Model file for the job. Use its own axes, mm. A direction names the side the tool comes from. Give positions to 0.01 mm unless a question says otherwise; leave off trailing zeros. Loops run counter-clockwise (first coordinate to the right, second up) from the corner with the lowest first, then second, coordinate; pieces in that order, holes last. Notation, with made-up numbers: M 47.25,12 L 52.25,12 A36 ccw 52.25,51 Z; hole C 55.25,84 d9. An arc over 180 degrees is marked long. Answer in a Markdown table with one row per item.
```python
from build123d import *

# Parameters (mm, degrees)
SKETCH1_R           = 173.85
SKETCH1_R_2         = 126.85
SKETCH1_R_3         = 4.1
BOSS_EXTRUDE1_DEPTH = 5
SKETCH1_3_R         = 146.85
SKETCH1_3_R_2       = 144.85
SKETCH1_3_R_3       = 126.85
BOSS_EXTRUDE2_DEPTH = 30
CUT_EXTRUDE1_START  = 9.5
SKETCH1_4_R         = 146.85
SKETCH1_4_R_2       = 144.85
CUT_EXTRUDE1_DEPTH  = 2.5
CUT_EXTRUDE2_START  = 21.5
SKETCH1_5_R         = 146.85
SKETCH1_5_R_2       = 144.85
CUT_EXTRUDE2_DEPTH  = 2.5


with BuildPart() as part:
    # Sketch1 → Boss-Extrude1 (new body)
    with BuildSketch(Plane(origin=(0, 0, 0), x_dir=(1, 0, 0), z_dir=(0, 1, 0))):
        with Locations(Location((0, 0, 0), (0, 0, 270))):
            Circle(SKETCH1_R)
        with Locations(Location((0, 0, 0), (0, 0, 270))):
            Circle(SKETCH1_R_2, mode=Mode.SUBTRACT)
        with Locations(Location((0, 161.925, 0), (0, 0, 270))):
            Circle(SKETCH1_R_3, mode=Mode.SUBTRACT)
        with Locations(Location((140.231163508, 80.9625, 0), (0, 0, 270))):
            Circle(SKETCH1_R_3, mode=Mode.SUBTRACT)
        with Locations(Location((140.231163508, -80.9625, 0), (0, 0, 270))):
            Circle(SKETCH1_R_3, mode=Mode.SUBTRACT)
        with Locations(Location((0, -161.925, 0), (0, 0, 270))):
            Circle(SKETCH1_R_3, mode=Mode.SUBTRACT)
        with Locations(Location((-140.231163508, -80.9625, 0), (0, 0, 270))):
            Circle(SKETCH1_R_3, mode=Mode.SUBTRACT)
        with Locations(Location((-140.231163508, 80.9625, 0), (0, 0, 270))):
            Circle(SKETCH1_R_3, mode=Mode.SUBTRACT)
    extrude(amount=BOSS_EXTRUDE1_DEPTH)

    # Sketch1_3 → Boss-Extrude2 (add)
    # profile 1 of 2: a face of its own
    with BuildSketch(Plane(origin=(0, 0, 0), x_dir=(1, 0, 0), z_dir=(0, 1, 0))):
        with Locations(Location((0, 0, 0), (0, 0, 270))):
            Circle(SKETCH1_3_R)
        Circle(SKETCH1_3_R_2, mode=Mode.SUBTRACT)
    # profile 2 of 2: a face of its own
    with BuildSketch(Plane(origin=(0, 0, 0), x_dir=(1, 0, 0), z_dir=(0, 1, 0))):
        Circle(SKETCH1_3_R_2)
        with Locations(Location((0, 0, 0), (0, 0, 270))):
            Circle(SKETCH1_3_R_3, mode=Mode.SUBTRACT)
    extrude(amount=BOSS_EXTRUDE2_DEPTH)

    # Sketch1_4 → Cut-Extrude1 (cut)
    with BuildSketch(Plane(origin=(0, 0, 0), x_dir=(1, 0, 0), z_dir=(0, 1, 0)).offset(CUT_EXTRUDE1_START)):
        with Locations(Location((0, 0, 0), (0, 0, 270))):
            Circle(SKETCH1_4_R)
        with Locations(Location((0, 0, 0), (0, 0, 270))):
            Circle(SKETCH1_4_R_2, mode=Mode.SUBTRACT)
    extrude(amount=CUT_EXTRUDE1_DEPTH, mode=Mode.SUBTRACT)

    # Sketch1_5 → Cut-Extrude2 (cut)
    with BuildSketch(Plane(origin=(0, 0, 0), x_dir=(1, 0, 0), z_dir=(0, 1, 0)).offset(CUT_EXTRUDE2_START)):
        with Locations(Location((0, 0, 0), (0, 0, 270))):
            Circle(SKETCH1_5_R)
        with Locations(Location((0, 0, 0), (0, 0, 270))):
            Circle(SKETCH1_5_R_2, mode=Mode.SUBTRACT)
    extrude(amount=CUT_EXTRUDE2_DEPTH, mode=Mode.SUBTRACT)


solid = part.part
```
(1) Saw through at B-B, the plane x = -43.5. Give the cut face in (y, z), and give its area (3 significant figures).
Established:
| item | result |
|---|---|
| outline | M 0,-168.32 L 5,-168.32 L 5,-140.26 L 9.5,-140.26 L 9.5,-138.16 L 12,-138.16 L 12,-140.26 L 21.5,-140.26 L 21.5,-138.16 L 24,-138.16 L 24,-140.26 L 30,-140.26 L 30,-119.16 L 0,-119.16 Z; M 0,119.16 L 30,119.16 L 30,140.26 L 24,140.26 L 24,138.16 L 21.5,138.16 L 21.5,140.26 L 12,140.26 L 12,138.16 L 9.5,138.16 L 9.5,140.26 L 5,140.26 L 5,168.32 L 0,168.32 Z |
| area | 1,530 mm2 |
(2) Saw through at A-A, the plane z = 0. Give the cut face in (x, y).
Established:
| item | result |
|---|---|
| outline | M -173.85,0 L -126.85,0 L -126.85,30 L -146.85,30 L -146.85,24 L -144.85,24 L -144.85,21.5 L -146.85,21.5 L -146.85,12 L -144.85,12 L -144.85,9.5 L -146.85,9.5 L -146.85,5 L -173.85,5 Z; M 126.85,0 L 173.85,0 L 173.85,5 L 146.85,5 L 146.85,9.5 L 144.85,9.5 L 144.85,12 L 146.85,12 L 146.85,21.5 L 144.85,21.5 L 144.85,24 L 146.85,24 L 146.85,30 L 126.85,30 Z |
(3) Mould opens along X. For faces 1 (the cylindrical face through (44.11, 7.22, 140.07)), 2 (the flat face through (-109.5, 30, 64.6)), 3 (the cylindrical face through (141.46, 2.46, -77.05)) say: pulls with the +X half, pulls with the -X half, needs draft (parallel to the pull), parting line crosses it, or undercut.
Established:
| item | result |
|---|---|
| face 1 | parting line crosses it |
| face 2 | needs draft |
| face 3 | undercut |
(4) Flat gauge pins, fed straight in: P1, Ø2, axis at y = 20, z = -135, coming from the +X side; P2, Ø7.5, axis at x = 0, z = 161.925, coming from the -Y side; P3, Ø1, axis at y = 8.5, z = 5.5, coming from the +X side; P4, Ø1.5, axis at y = 5.5, z = -104, coming from the +X side. Where does each tip first touch, or does it go through?
Established:
| item | result |
|---|---|
| P1 | stops at x = 60.07 |
| P2 | passes through |
| P3 | stops at x = 146.76 |
| P4 | stops at x = 139.73 |
(5) Wall check: L1, parallel to X at y = 11.25, z = -4.5; L2, parallel to Z at x = -27, y = 14.75; L3, parallel to Z at x = -21.5, y = 24.5. Give the ranges that are in metal, low to high.
Established:
| item | result |
|---|---|
| L1 | x = -144.78 to -126.77, 126.77 to 144.78 |
| L2 | z = -144.35 to -123.94, 123.94 to 144.35 |
| L3 | z = -145.27 to -125.01, 125.01 to 145.27 |
(6) Which spindle directions (+Z, -Z, +X, -X, +Y, -Y) get a long thin tool onto all of the face, cutting with end or side? Do faces 4 (the flat face through (-97, 21.5, 108)), 5 (the cylindrical face through (-77.19, 14.79, -100.66)), 6 (the cylindrical face through (44.11, 26.96, 140.07)). Say none if no direction does.
Established:
| item | result |
|---|---|
| face 4 | none |
| face 5 | +Y, -Y |
| face 6 | +Y |
(7) Saw through at C-C, the plane x = 0. Count the separate pieces of the cut face and the enclosed holes in it, and give its area (3 significant figures).
Established:
| item | result |
|---|---|
| separate pieces | 4 |
| enclosed holes | 0 |
| area | 1,370 mm2 |
